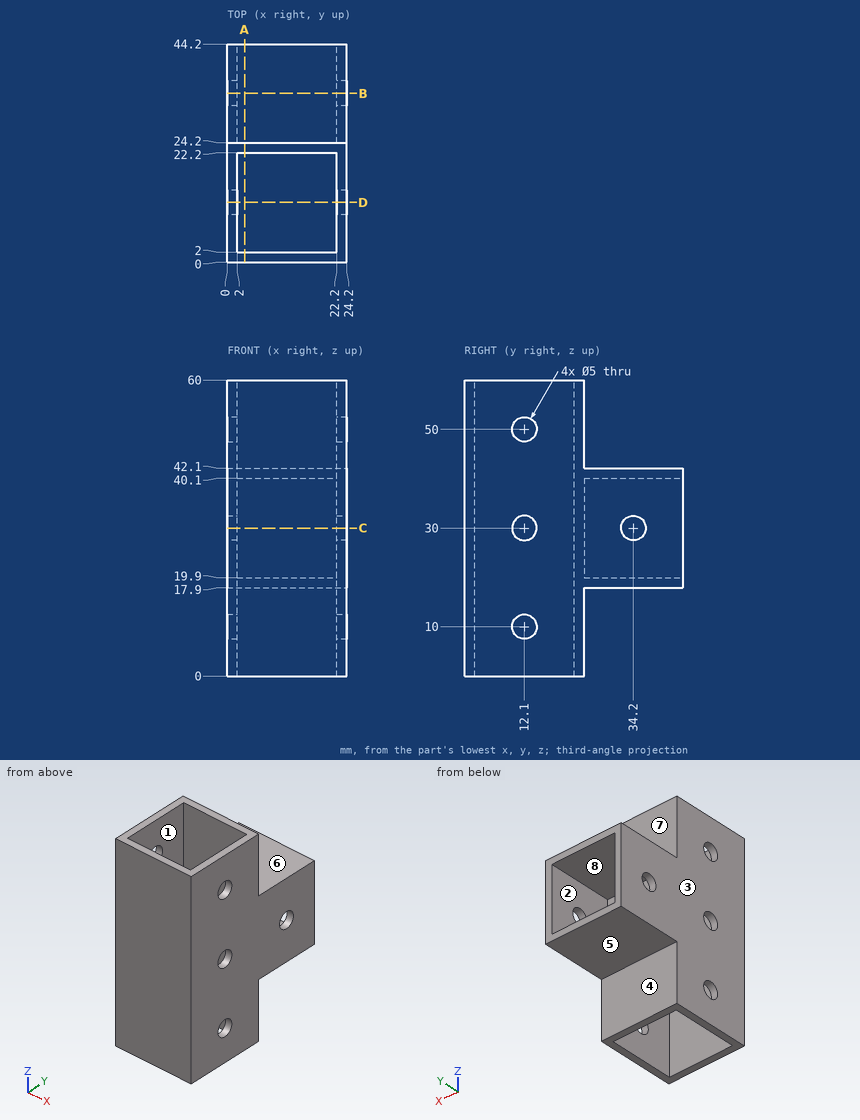
Geometry check sheet. Reference: drawing and pictorial views, mm from the part's lowest x, y, z. A direction names the side the tool comes from. Give positions to 0.01 mm unless a question says otherwise; leave off trailing zeros. Order: outer loops, then holes, each group sorted by start corner. A loop starts at its lowest first (then second) coordinate and runs counter-clockwise, first axis right, second up. Notation, with made-up numbers: M -36,66 L -24,66 A29 cw -24,103 Z; hole C 17,-21 d4. An arc over 180 degrees is marked long. Answer as a JSON object with one key per item and string values. Group by question number.
1) Cross-section at C-C (z = 30). Enter the section's corners in (x, y), then the cut area to 3 significant figures.
2) Cross-section at B-B (y = 34.2). Enter the section's corners in (x, z), then the cut area to 3 significant figures.
3) Mould release check, pull along Z, two halves, no side actions. Record for the marked faces 5, 6, 7 and 8: released by +Z, released by -Z, zero draft, split by the parting line, or undercut.
4) Depth check by flat-ended pin: pin 1 Ø2 at (x, z) = (10.5, 23) entering from +Y; pin 2 Ø6 at (x, y) = (12, 30.5) entering from -Z. Enter the tip coordinate at first touch or a pass-through.
5) Cross-section at D-D (y = 12.1). Give the number of separate pieces and of enclosed holes in the cut face, then the cut area to 3 significant figures.
6) Access from +Z, -Z, +X, -X, +Y, -Y to the whole of each face (thin tool, end or side, straight path). Record for the marked faces 1, 2, 3 and 4.
7) Scan lines: line 1 along Y through (x, z) = (0.7, 30); line 2 along Y through (x, z) = (3, 38). Record each from-to range of solid material in increasing order. Write a range as [from, to].
8) Cross-section at A-A (x = 3.5). Enter the section's corners in (y, z).
Result sheet:
{
 "1": {"outline": "M 0,0 L 24.2,0 L 24.2,9.6 L 22.2,9.6 L 22.2,2 L 2,2 L 2,9.6 L 0,9.6 Z; M 0,14.6 L 2,14.6 L 2,22.2 L 22.2,22.2 L 22.2,14.6 L 24.2,14.6 L 24.2,31.7 L 22.2,31.7 L 22.2,24.2 L 2,24.2 L 2,31.7 L 0,31.7 Z; M 0,36.7 L 2,36.7 L 2,44.2 L 0,44.2 Z; M 22.2,36.7 L 24.2,36.7 L 24.2,44.2 L 22.2,44.2 Z", "area": "218 mm2"},
 "2": {"outline": "M 0,17.9 L 24.2,17.9 L 24.2,27.5 L 22.2,27.5 L 22.2,19.9 L 2,19.9 L 2,27.5 L 0,27.5 Z; M 0,32.5 L 2,32.5 L 2,40.1 L 22.2,40.1 L 22.2,32.5 L 24.2,32.5 L 24.2,42.1 L 0,42.1 Z", "area": "158 mm2"},
 "3": {"face 5": "released by -Z", "face 6": "released by +Z", "face 7": "zero draft", "face 8": "undercut"},
 "4": {"pin 1": "stops at y = 24.2", "pin 2": "stops at z = 17.9"},
 "5": {"separate pieces": "8", "enclosed holes": "0", "area": "180 mm2"},
 "6": {"face 1": "+Z, -Z", "face 2": "+Y", "face 3": "+Z, -Z, -X, +Y, -Y", "face 4": "-Z, +X, -X, +Y"},
 "7": {"line 1": "y = [0, 9.6], [14.6, 31.7], [36.7, 44.2]", "line 2": "y = [0, 2], [22.2, 24.2]"},
 "8": {"outline": "M 0,0 L 2,0 L 2,60 L 0,60 Z; M 22.2,0 L 24.2,0 L 24.2,17.9 L 44.2,17.9 L 44.2,19.9 L 24.2,19.9 L 24.2,40.1 L 44.2,40.1 L 44.2,42.1 L 24.2,42.1 L 24.2,60 L 22.2,60 Z"}
}
